Autodesk Inventor part; units mm, degrees
ref_plane "YZ Plane" through (0, 0, 0) normal (1, 0, 0) x (0, 1, 0)
ref_plane "XZ Plane" through (0, 0, 0) normal (0, 1, 0) x (-1, 0, 0)
ref_plane "XY Plane" through (0, 0, 0) normal (0, 0, 1) x (1, 0, 0)
sketch "Sketch1" plane through (0, 0, 0) normal (1, 0, 0) x (0, 1, 0)
  circle A0 centre (0, 0) radius 5
  dimension "d0" = 10
extrude "Extrusion1" add sketch "Sketch1" along normal blind 52.5
sketch "Sketch2" plane through (52.5, 0, 0) normal (1, 0, 0) x (0, 0, -1)
  circle A0 centre (0, 0) radius 1.5
  dimension "d3" = 3
extrude "Extrusion2" add sketch "Sketch2" along normal blind 11.5
sketch "Sketch3" plane through (64, 0, 0) normal (1, 0, 0) x (0, 0, -1)
  circle A0 centre (0, 0) radius 5
  dimension "d6" = 10
extrude "Extrusion3" add sketch "Sketch3" along normal blind 1
sketch "Sketch4" plane through (65, 0, 0) normal (1, 0, 0) x (0, 0, -1)
  circle A0 centre (0, 0) radius 3.75
  dimension "d9" = 7.5
extrude "Extrusion4" add sketch "Sketch4" along normal blind 8
sketch "Sketch5" plane through (73, 0, 0) normal (1, 0, 0) x (0, 0, -1)
  circle A0 centre (0, 0) radius 1.5
  dimension "d12" = 3
extrude "Extrusion5" cut sketch "Sketch5" against normal blind 8
sketch "Sketch6" plane through (0, 0, 0) normal (-1, 0, 0) x (0, 0, 1)
  circle A0 centre (0, 0) radius 3.75
  circle A1 centre (0, 0) radius 4.5
  circle A2 centre (0, 0) radius 1.5
  circle A3 centre (0, 0) radius 5
  dimension "d15" = 9
  dimension "d16" = 10
extrude "Extrusion6" cut sketch "Sketch6" against normal blind 10.5 contours A3
sketch "Sketch7" plane through (10.5, 0, 0) normal (-1, 0, 0) x (0, 0, 1)
  circle A0 centre (0, 0) radius 8.5
  dimension "d19" = 17
extrude "Extrusion7" add sketch "Sketch7" along normal blind 1
sketch "Sketch8" plane through (0, 0, 0) normal (-1, 0, 0) x (0, 0, 1)
  line L0 (-6, 1.5) -> (6, 1.5)
  line L1 (6, 1.5) -> (6, -1.5)
  line L2 (6, -1.5) -> (-6, -1.5)
  line L3 (-6, -1.5) -> (-6, 1.5)
  line L4 (-6, 1.5) -> (6, -1.5) construction
  line L5 (6, 1.5) -> (-6, -1.5) construction
  point P0 (0, 0)
  point P1 (0, 0)
  dimension "d23" = 12
extrude "Extrusion8" cut sketch "Sketch8" against normal blind 9
sketch "Sketch10" plane through (9.5, 0, 0) normal (-1, 0, 0) x (0, 0, 1)
  circle A0 centre (0, 0) radius 6
  circle A1 centre (0, 0) radius 1.5
  circle A2 centre (0, 0) radius 4.8442
extrude "Extrusion10" add sketch "Sketch10" along normal blind 9.5 contours A0
sketch "Sketch12" plane through (0, 0, 0) normal (-1, 0, 0) x (0, 0, 1)
  line L0 (-8.4132, -1.5) -> (8.4132, -1.5)
  line L1 (8.4132, -1.5) -> (8.4132, 1.5)
  line L2 (8.4132, 1.5) -> (-8.4132, 1.5)
  line L3 (-8.4132, 1.5) -> (-8.4132, -1.5)
  line L4 (-8.4132, -1.5) -> (8.4132, 1.5) construction
  line L5 (8.4132, -1.5) -> (-8.4132, 1.5) construction
  point P0 (0, 0)
  dimension "d35" = 3
extrude "Extrusion12" cut sketch "Sketch12" against normal blind 9
sketch "Sketch13" plane through (0, 1.5, -5.8095) normal (0, -1, 0) x (1, 0, 0)
  line L0 (-3.5, 6.3202) -> (3.5, 6.3202)
  line L1 (3.5, 6.3202) -> (3.5, 5.2988)
  line L2 (3.5, 5.2988) -> (-3.5, 5.2988)
  line L3 (-3.5, 5.2988) -> (-3.5, 6.3202)
  line L4 (-3.5, 6.3202) -> (3.5, 5.2988) construction
  line L5 (3.5, 6.3202) -> (-3.5, 5.2988) construction
  circle A0 centre (3.5, 5.8095) radius 1.5
  point P0 (0, 5.8095)
  dimension "d38" = 7
  dimension "d39" = 3
extrude "Extrusion13" cut sketch "Sketch13" along normal through all both and the other way through all contours A0 L2 L1 L0 | L0 L1 L2 A0
properties part number "shaft"
Source: CAD feature listing. Evaluate the final solid. Frame: model axes, mm. A direction names the side the tool comes from. Coordinates: 2 decimals unless noted, no trailing zeros. Loops run counter-clockwise (first coordinate to the right, second up) from the corner with the lowest first, then second, coordinate; pieces in that order, holes last. Notation, with made-up numbers: M 10.25,-12.5 L 52.25,-12.5 A16 ccw 52.25,9.5 Z; hole C 76,55 d8. An arc over 180 degrees is marked long. Use CSV: the item, a comma, the result in double quotes.
(1) Cut plane B-B on x = 44. Return loops of the section in (y, z), and give its area (3 significant figures).
Answers follow:
outline,"C 0,0 d10"
area,"78.5 mm²"
(2) Line query: line 1 (X direction, y = 3.4, z = 0); line 2 (X direction, y = 3, z = -3); line 3 (Y direction, x = 7, z = -1). Output: solid intervals per line, ascending. Write a range as [from, to].
Answers follow:
line 1,"[0, 2], [5, 52.5], [64, 73]"
line 2,"[0, 52.5], [64, 65]"
line 3,"[-5.92, -4.74], [-4.39, -1.5], [1.5, 4.39], [4.74, 5.92]"
(3) Cut plane A-A on x = 3.5. Return loops of the section in (y, z).
Answers follow:
outline,"M -5.81,-1.5 A6 ccw -1.5,-5.81 L -1.5,-4.61 A4.84 cw -4.61,-1.5 Z; M -5.81,1.5 L -4.61,1.5 A4.84 cw -1.5,4.61 L -1.5,5.81 A6 ccw Z; M -4.24,-1.5 A4.5 ccw -1.5,-4.24 L -1.5,-1.5 Z; M -4.24,1.5 L -1.5,1.5 L -1.5,4.24 A4.5 ccw Z; M 1.5,-5.81 A6 ccw 5.81,-1.5 L 4.61,-1.5 A4.84 cw 1.5,-4.61 Z; M 1.5,-4.24 A4.5 ccw 4.24,-1.5 L 1.5,-1.5 Z; M 1.5,1.5 L 4.24,1.5 A4.5 ccw 1.5,4.24 Z; M 1.5,4.61 A4.84 cw 4.61,1.5 L 5.81,1.5 A6 ccw 1.5,5.81 Z"
(4) Cut plane C-C on z = 7.25. Return loops of the section in (x, y).
Answers follow:
outline,"M 9.5,-4.44 L 10.5,-4.44 L 10.5,4.44 L 9.5,4.44 Z"
(5) Reachability of faces 4 (the face through (0, -3, 0)), 5 (the face through (65, 4, -1)), 6 (the face through (64, 1.2, 1.2)), 7 (the face through (4.19, 5.29, -1.33)), 8 (the face through (9, 0, 0)) from +Z, -Z, +X, -X, +Y, -Y: full face, straight path, thin tool, end or side. Return the list, or none.
Answers follow:
face 4,"+Z, -Z, -X, +Y, -Y"
face 5,"+X"
face 6,"none"
face 7,"+Y, -Y"
face 8,"+Z, -Z, -X"
(6) Draft query along X for faces 1 (the face through (0, -5, 0)), 2 (the face through (4.886, -5.313, -0.575)), 3 (the face through (4, -1.5, -5)). Return one class per face: pulls with the +X half, pulls with the -X half, needs draft (parallel to the pull), parting line crosses it, or undercut.
Answers follow:
face 1,"pulls with the -X half"
face 2,"undercut"
face 3,"needs draft"
(7) Contact query for flat-ended pins moving along their axis: pin 1 (4 mm diameter, centred on x = 6.5, z = -0.5, fed in from +Y); pin 2 (5 mm diameter, centred on x = 3.5, z = 0, fed in from -Y); pin 3 (1.5 mm diameter, centred on y = 0.5, z = 5.5, fed in from -X). Output: stop coordinate, or through.
Answers follow:
pin 1,"y = 6"
pin 2,"y = -6"
pin 3,"x = 9"
(8) Cut plane D-D on y = -7. Return loops of the section in (x, z), and give its area (3 significant figures).
Answers follow:
outline,"M 9.5,-4.82 L 10.5,-4.82 L 10.5,4.82 L 9.5,4.82 Z"
area,"9.64 mm²"
